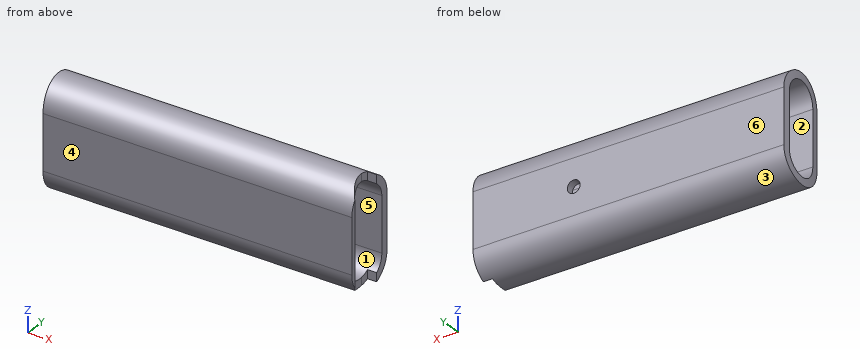
```python
from build123d import *

# Parameters (mm, degrees)
EXTRUSION1_DEPTH             = 51
ENL_V_MAT_EXTRU_2_DEPTH      = 18.5
ENL_V_MAT_EXTRU_2_DEPTH_BACK = 18.5
ENL_V_MAT_EXTRU_3_REACH      = 19
ESQUISSE4_R                  = 2.1
ENL_V_MAT_EXTRU_4_DEPTH      = 18.5000001
ENL_V_MAT_EXTRU_4_DEPTH_BACK = 18.5000001


with BuildPart() as part:
    # Esquisse1 → Extrusion1 (new body, symmetric)
    with BuildSketch(Plane(origin=(0, 0, 0), x_dir=(0, 0, -1), z_dir=(1, 0, 0))):
        with BuildLine():
            Line((-9, -8.5), (9, -8.5))
            ThreePointArc((9, -8.5), (17.5, 0), (9, 8.5))
            Line((9, 8.5), (-9, 8.5))
            ThreePointArc((-9, 8.5), (-17.5, 0), (-9, -8.5))
        make_face()
        with BuildLine():
            Line((-9, 6), (9, 6))
            ThreePointArc((9, 6), (15, 0), (9, -6))
            Line((9, -6), (-9, -6))
            ThreePointArc((-9, -6), (-15, 0), (-9, 6))
        make_face(mode=Mode.SUBTRACT)
    extrude(amount=EXTRUSION1_DEPTH, both=True)

    # Esquisse3 → Enlèv. mat.-Extru.2 (cut, two sides)
    with BuildSketch(Plane.XY) as enl_v_mat_extru_2_sk:
        with BuildLine():
            Line((51, 3.5), (48, 3.5))
            Line((48, 3.5), (48, 0.5))
            ThreePointArc((48, 0.5), (48.77747585, -3.562019202), (51, -7.049834435))
            Line((51, -7.049834435), (51, 3.5))
        make_face()
    extrude(amount=ENL_V_MAT_EXTRU_2_DEPTH, mode=Mode.SUBTRACT)
    extrude(enl_v_mat_extru_2_sk.sketch, amount=-ENL_V_MAT_EXTRU_2_DEPTH_BACK, mode=Mode.SUBTRACT)

    # Esquisse4 → Enlèv. mat.-Extru.3 (cut, up to next)
    with BuildSketch(Plane(origin=(0, 8.5, 0), x_dir=(-1, 0, 0), z_dir=(0, 1, 0)), mode=Mode.PRIVATE) as enl_v_mat_extru_3_sk1:
        with Locations(Location((-18, 0, 0), (0, 0, 90))):  # turned: the seam where the file's is
            Circle(ESQUISSE4_R)
    enl_v_mat_extru_3_tool1 = extrude(enl_v_mat_extru_3_sk1.sketch, amount=-ENL_V_MAT_EXTRU_3_REACH, mode=Mode.PRIVATE) & part.part
    add(enl_v_mat_extru_3_tool1.solids().sort_by_distance((18, 8.5, 0))[0], mode=Mode.SUBTRACT)

    # Esquisse5 → Enlèv. mat.-Extru.4 (cut, two sides)
    with BuildSketch(Plane.XY) as enl_v_mat_extru_4_sk:
        with BuildLine():
            Line((60.682276478, -226.426742354), (-41.324705982, -35.5))
            ThreePointArc((-41.324705982, -35.5), (-49.153043001, -14.164640947), (-50.824705982, 8.5))
            Line((-50.824705982, 8.5), (-36.678065011, 224.505365595))
            Line((-36.678065011, 224.505365595), (-459.862900179, 133.135912547))
            Line((-459.862900179, 133.135912547), (-362.50255869, -317.796195402))
            Line((-362.50255869, -317.796195402), (60.682276478, -226.426742354))
        make_face()
    extrude(amount=ENL_V_MAT_EXTRU_4_DEPTH, mode=Mode.SUBTRACT)
    extrude(enl_v_mat_extru_4_sk.sketch, amount=-ENL_V_MAT_EXTRU_4_DEPTH_BACK, mode=Mode.SUBTRACT)


solid = part.part
```
Here's how the part is built. I have some questions about the finished solid (model axes, mm). Face numbers are marked on the shaded views. A direction names the side the tool comes from. Give positions to 0.01 mm unless a question says otherwise; leave off trailing zeros. Loops run counter-clockwise (first coordinate to the right, second up) from the corner with the lowest first, then second, coordinate; pieces in that order, holes last. Notation, with made-up numbers: M 39.25,-37.5 L 56.25,-37.5 A16 cw 56.25,-27.5 Z; hole C 50,-12 d8. An arc over 180 degrees is marked long. Put each result on its own line as item: value. Start each with the question number.
(1) Will these pins go through, and if not, where does the flat tip stop? pin 1 Ø1.5 at (y, z) = (-4.5, 0.5) entering from -X; pin 2 Ø1 at (x, z) = (-25.5, -14) entering from +Y; pin 3 Ø3 at (x, y) = (19.5, 2) entering from +Z; pin 4 Ø1 at (y, z) = (-6.5, -12.5) entering from +X.
(2) I want a section at A-A on z = 0. Please give me the cut outline in (x, y), then the cut area to 3 significant figures.
(3) I want a section at D-D on y = -3.25. Please give me the cut outline in (x, z).
(4) I want a section at B-B on z = -4. Please give me the cut outline in (x, y).
(5) I need wall thicknesses on line 1 along Y through (x, z) = (-10, 9.5); line 2 along Z through (x, y) = (-19, -0.5); line 3 along X through (y, z) = (6.65, 0). Which ranges of each line are inside material? Lowest first, please. Write a range as [from, to].
(6) I want a section at C-C on x = 18. Please give me the cut outline in (y, z).
(7) For the marked faces 5 and 6, which set-ups out of +Z, -Z, +X, -X, +Y, -Y let a thin tool reach every point of the face, with its end or its side?
(8) If we mould it in two halves opening along Z, with no side actions, what happens to the marked faces 1, 2, 3 and 4? For each: +Z half, -Z half, draft (parallel to the pull), parting line (faces both ways), or undercut.
Answer block:
1. pin 1: through
1. pin 2: y = 7.21
1. pin 3: z = 17.49
1. pin 4: x = 50.95
2. outline: M -50.95,6 L 15.9,6 L 15.9,8.5 L -50.82,8.5 A82 ccw Z; M -50.49,-6 A82 ccw -50.17,-8.5 L 51,-8.5 L 51,-7.05 A11 cw 50.13,-6 Z; M 20.1,6 L 51,6 L 51,8.5 L 20.1,8.5 Z
2. area: 497 mm^2
3. outline: M -50.75,-16.85 L 48.66,-16.85 L 48.66,-14.04 L -50.75,-14.04 Z; M -50.75,14.04 L 48.66,14.04 L 48.66,16.85 L -50.75,16.85 Z
4. outline: M -50.95,6 L 51,6 L 51,8.5 L -50.82,8.5 A82 ccw Z; M -50.49,-6 A82 ccw -50.17,-8.5 L 51,-8.5 L 51,-7.05 A11 cw 50.13,-6 Z
5. line 1: [-8.49, -5.98], [5.98, 8.49]
5. line 2: [-17.49, -14.98], [14.98, 17.49]
5. line 3: [-50.92, 15.9], [20.1, 51]
6. outline: M -8.5,-9 A8.5 ccw 8.5,-9 L 8.5,-2.1 L 6,-2.1 L 6,-9 A6 cw -6,-9 L -6,9 A6 cw 6,9 L 6,2.1 L 8.5,2.1 L 8.5,9 A8.5 ccw -8.5,9 Z
7. face 5: +X, -X
7. face 6: +Z, -Z, +X, -X, +Y
8. face 1: undercut
8. face 2: undercut
8. face 3: -Z half
8. face 4: draft
